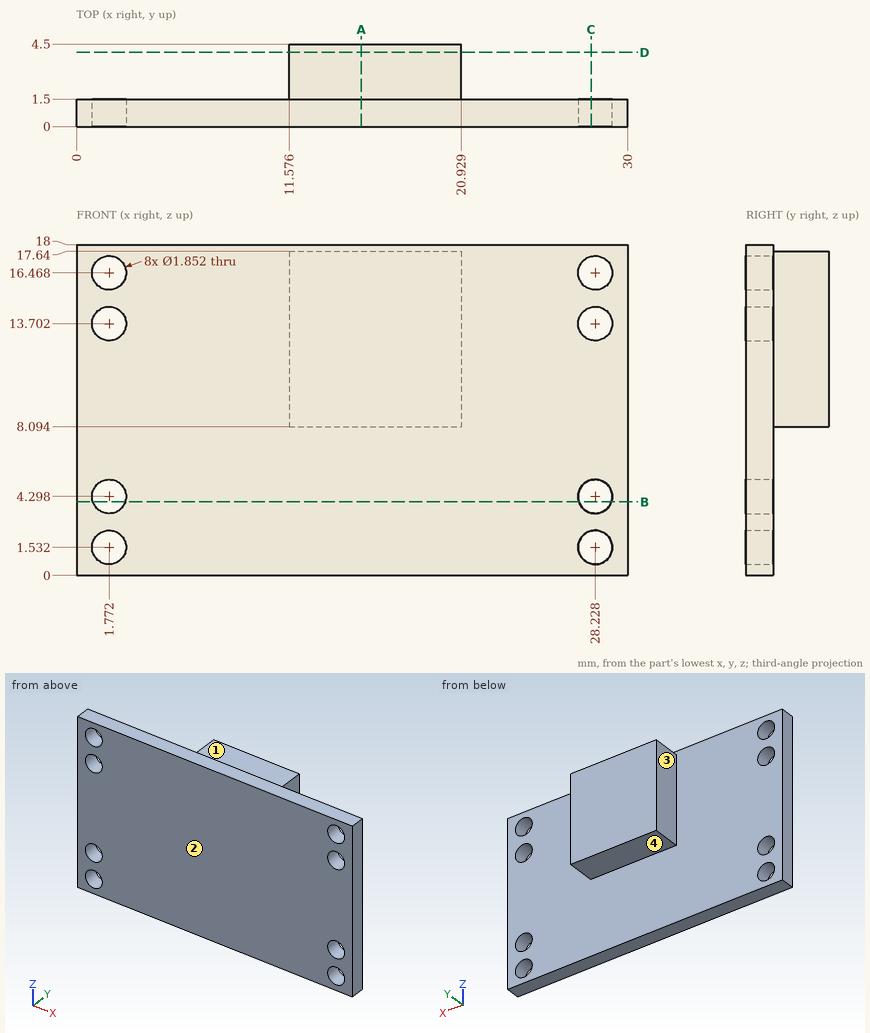
Geometry: see drawing. Coordinates: mm, zero at the bounding-box minimum. A direction names the side the tool comes from. Give positions to 0.01 mm unless a question says otherwise; leave off trailing zeros. Write each loop counter-clockwise with the first axis right and the second up, starting at its lowest first coordinate (ties: lowest second). Pieces come first, ordered by that corner, then holes. Notation, with made-up numbers: M 35.25,69 L 40.25,69 A11 cw 40.25,85 Z; hole C 49,9.5 d1. An arc over 180 degrees is marked long. Return JSON: item names as keys, results as strings. Group by question number.
1) Cut plane D-D, the plane y = 4.05. Output: boundary loops of the cut face in (x, z) (1 decimal).
2) Cut plane B-B, the plane z = 4. Output: boundary loops of the cut face in (x, y) (1 decimal).
3) First-contact query: pin 1 Ø1.5 at (y, z) = (2.5, 8.5) entering from -X; pin 2 Ø0.9 at (x, y) = (18, 3.5) entering from +Z; pin 3 Ø3 at (x, z) = (28.23, 4.3) entering from +Y. Flat tips, straight axial feed; report the tip coordinate or a pass-through.
4) Ray query, L1, parallel to Y at x = 8.75, z = 5; L2, parallel to Z at x = 28, y = 1.1 (1 decimal); L3, parallel to X at y = 3.6, z = 16.75 (1 decimal). Return the intervals inside material, ascending.
5) Set-up query: the marked faces 1, 2, 3 and 4. Return all of +Z, -Z, +X, -X, +Y, -Y with unobstructed straight access to the full face (end or side cutting, diameter ignored); none if empty.
6) Cut plane A-A, the plane x = 15.5. Output: boundary loops of the cut face in (y, z).
7) Cut plane C-C, the plane x = 28. Output: boundary loops of the cut face in (y, z) (1 decimal).
Data:
{
 "1": {"outline": "M 11.6,8.1 L 20.9,8.1 L 20.9,17.6 L 11.6,17.6 Z"},
 "2": {"outline": "M 0,0 L 0.9,0 L 0.9,1.5 L 0,1.5 Z; M 2.6,0 L 27.4,0 L 27.4,1.5 L 2.6,1.5 Z; M 29.1,0 L 30,0 L 30,1.5 L 29.1,1.5 Z"},
 "3": {"pin 1": "stops at x = 11.58", "pin 2": "stops at z = 17.64", "pin 3": "stops at y = 1.5"},
 "4": {"L1": "y = 0 to 1.5", "L2": "z = 0 to 0.6, 2.4 to 3.4, 5.2 to 12.8, 14.6 to 15.6, 17.4 to 18", "L3": "x = 11.6 to 20.9"},
 "5": {"face 1": "+Z, +X, -X, +Y", "face 2": "+Z, -Z, +X, -X, -Y", "face 3": "+Z, -Z, -X, +Y", "face 4": "-Z, +X, -X, +Y"},
 "6": {"outline": "M 0,0 L 1.5,0 L 1.5,8.09 L 4.5,8.09 L 4.5,17.64 L 1.5,17.64 L 1.5,18 L 0,18 Z"},
 "7": {"outline": "M 0,0 L 1.5,0 L 1.5,0.6 L 0,0.6 Z; M 0,2.4 L 1.5,2.4 L 1.5,3.4 L 0,3.4 Z; M 0,5.2 L 1.5,5.2 L 1.5,12.8 L 0,12.8 Z; M 0,14.6 L 1.5,14.6 L 1.5,15.6 L 0,15.6 Z; M 0,17.4 L 1.5,17.4 L 1.5,18 L 0,18 Z"}
}
